```python
from build123d import *

# Parameters (mm, degrees)
SKETCH1_W                 = 25.4
SKETCH1_H                 = 19.05
SKETCH1_R                 = 2.1463
BOSS_EXTRUDE1_DEPTH       = 6.35
F_4_40_TAPPED_HOLE1_D     = 2.2606
F_4_40_TAPPED_HOLE1_DEPTH = 7.5946
F_4_40_TAPPED_HOLE1_TIP   = 0.679152758
FILLET1_R                 = 6.35


with BuildPart() as part:
    # Sketch1 → Boss-Extrude1 (new body)
    with BuildSketch(Plane(origin=(0, 0, 0), x_dir=(1, 0, 0), z_dir=(0, 1, 0))):
        with Locations((6.35, 0)):
            Rectangle(SKETCH1_W, SKETCH1_H)
        Circle(SKETCH1_R, mode=Mode.SUBTRACT)
    extrude(amount=BOSS_EXTRUDE1_DEPTH)

    # #4-40 Tapped Hole1
    with Locations(Plane(origin=(0, 6.35, 0), x_dir=(1, 0, 0), z_dir=(0, 1, 0))):
        with Locations((2.54, 5.715), (15.24, -5.715), (2.54, -5.715), (15.24, 5.715)):
            Hole(F_4_40_TAPPED_HOLE1_D / 2, depth=F_4_40_TAPPED_HOLE1_DEPTH)
            with Locations((0, 0, -(F_4_40_TAPPED_HOLE1_DEPTH + F_4_40_TAPPED_HOLE1_TIP / 2))):  # 118° drill point
                Cone(0, F_4_40_TAPPED_HOLE1_D / 2, F_4_40_TAPPED_HOLE1_TIP, mode=Mode.SUBTRACT)

    # Fillet1
    fillet1_edges = [part.edges().sort_by_distance(p)[0] for p in [
        (-6.35, 3.175, -9.525),
        (-6.35, 3.175, 9.525),
    ]]
    fillet(fillet1_edges, radius=FILLET1_R)


solid = part.part
```
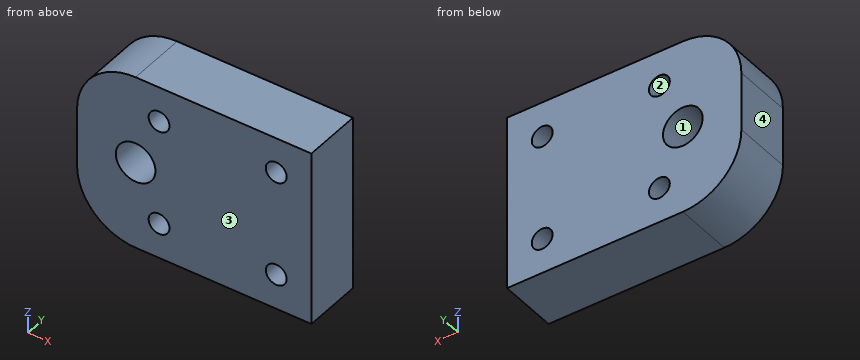
Work out the finished part from the listing and answer in its coordinate system (mm). Face numbers are marked on the shaded views. Coordinates: 2 decimals unless noted, no trailing zeros. Write each loop counter-clockwise with the first axis right and the second up, starting at its lowest first coordinate (ties: lowest second). Pieces come first, ordered by that corner, then holes.
Q1. A cutting plane is placed at D-D, the plane y = 4.75. Give the vertices of the cut face in (x, z) (3 decimals).
Q2. A cutting plane is placed at C-C, the plane z = 6.25. Give the vertices of the cut face in (x, y).
Q3. This flat-tipped pin is pushed along its axis until it touches: pin 1 Ø2 at (y, z) = (5.5, 7) entering from -X. Where does it stop, or does it pass through?
Q4. Determine the mould class of the marked faces 1, 2, 3 and 4 for opening direction X: released by +X, released by -X, zero draft, split by the parting line, or undercut.
Q5. A cutting plane is placed at B-B, the plane x = 15.24. Give the vertices of the cut face in (y, z) (3 decimals), then the cut area to 3 significant figures.
Q6. A cutting plane is placed at A-A, the plane z = 0. Give the vertices of the cut face in (x, y), then the cut area to 3 significant figures.
Q7. Find the intervals of material crossed by line 1 (Z direction, x = 15.24, y = 3) (3 decimals); line 2 (X direction, y = 1, z = -6.25); line 3 (X direction, y = 3, z = -6), in increasing order.
Findings below:
1. outline: (-6.35, -3.175) arc R6.35 ccw to (0, -9.525) - (19.05, -9.525) - (19.05, 9.525) - (0, 9.525) arc R6.35 ccw to (-6.35, 3.175) - close; hole circle Ø4.293 at (0, 0); hole circle Ø2.261 at (2.54, -5.715); hole circle Ø2.261 at (2.54, 5.715); hole circle Ø2.261 at (15.24, -5.715); hole circle Ø2.261 at (15.24, 5.715)
2. outline: (-5.56, 0) - (1.54, 0) - (1.54, 6.35) - (-5.56, 6.35) - close; (3.54, 0) - (14.24, 0) - (14.24, 6.35) - (3.54, 6.35) - close; (16.24, 0) - (19.05, 0) - (19.05, 6.35) - (16.24, 6.35) - close
3. pin 1: stops at x = -5.69
4. face 1: undercut
4. face 2: undercut
4. face 3: zero draft
4. face 4: released by -X
5. outline: (0, -9.525) - (6.35, -9.525) - (6.35, -6.845) - (0, -6.845) - close; (0, -4.585) - (6.35, -4.585) - (6.35, 4.585) - (0, 4.585) - close; (0, 6.845) - (6.35, 6.845) - (6.35, 9.525) - (0, 9.525) - close
5. area: 92.3 mm2
6. outline: (-6.35, 0) - (-2.15, 0) - (-2.15, 6.35) - (-6.35, 6.35) - close; (2.15, 0) - (19.05, 0) - (19.05, 6.35) - (2.15, 6.35) - close
6. area: 134 mm2
7. line 1: z = -9.525 to -6.845, -4.585 to 4.585, 6.845 to 9.525
7. line 2: x = -5.56 to 1.54, 3.54 to 14.24, 16.24 to 19.05
7. line 3: x = -5.69 to 1.45, 3.63 to 14.15, 16.33 to 19.05
